Autodesk Fusion 360 part; units mm, degrees
sketch "Sketch3" plane through (0, 0, 0) normal (0, 0, 1) x (1, 0, 0)
  line L0 (90, 40) -> (-90, 40)
  line L1 (-90, 40) -> (-90, -40)
  line L2 (-90, -40) -> (90, -40)
  line L3 (90, -40) -> (90, 40)
  line L4 (90, 40) -> (-90, -40) construction
  line L5 (-90, 40) -> (90, -40) construction
  line L6 (-92, -42) -> (92, -42)
  line L7 (92, -42) -> (92, 42)
  line L8 (92, 42) -> (-92, 42)
  line L9 (-92, 42) -> (-92, -42)
  dimension "d6" = 180
  dimension "d7" = 80
  dimension "d8" = 2
extrude "Extrude2" add sketch "Sketch3" along normal blind 5
extrude "Extrude3" add sketch "Sketch3" along normal blind 4 contours L0 L1 L2 L3
sketch "Sketch6" plane through (0, 0, 5) normal (0, 0, 1) x (-1, 0, 0)
  line L0 (-90, -40) -> (-90, 40)
  line L1 (-90, 40) -> (90, 40)
  line L2 (90, 40) -> (90, -40)
  line L3 (90, -40) -> (-90, -40)
  line L4 (92, -42) -> (92, 42)
  line L5 (92, 42) -> (-92, 42)
  line L6 (-92, 42) -> (-92, -42)
  line L7 (-92, -42) -> (92, -42)
  line L8 (-22, -27) -> (-22, -57)
  line L9 (22, -57) -> (22, -27)
  line L10 (22, -42) -> (-22, -42)
  line L11 (-22, -42) -> (-22, -72)
  line L12 (-22, -72) -> (22, -72)
  line L13 (22, -72) -> (22, -42)
  line L14 (22, -42) -> (-22, -72) construction
  line L15 (-22, -42) -> (22, -72) construction
  point P0 (0, -42)
  point P1 (0, -57)
  dimension "d20" = 44
  dimension "d21" = 30
  dimension "d22" = 44
  dimension "d23" = 30
extrude "Extrude4" add sketch "Sketch6" against normal blind 5 contours L7 L8 L9 L10 L11 L12 L13
sketch "Sketch7" plane through (0, 0, 5) normal (0, 0, 1) x (-1, 0, 0)
  line L0 (-90, -40) -> (-90, 40)
  line L1 (-90, 40) -> (90, 40)
  line L2 (90, 40) -> (90, -40)
  line L3 (90, -40) -> (-90, -40)
  line L4 (92, -42) -> (92, 42)
  line L5 (92, 42) -> (-92, 42)
  line L6 (-92, 42) -> (-92, -42)
  line L7 (-92, -42) -> (-22, -42)
  line L8 (-22, -42) -> (-22, -72)
  line L9 (-22, -72) -> (22, -72)
  line L10 (22, -72) -> (22, -42)
  line L11 (22, -42) -> (92, -42)
  circle A0 centre (-18, -68) radius 1.5
  circle A1 centre (18, -68) radius 1.5
  circle A2 centre (-18, -47) radius 1.5
  circle A3 centre (18, -47) radius 1.5
  dimension "d26" = 3
  dimension "d27" = 4
  dimension "d28" = 4
  dimension "d29" = 3
  dimension "d30" = 3
  dimension "d31" = 3
  dimension "d32" = 4
  dimension "d33" = 4
  dimension "d34" = 4
  dimension "d35" = 7
  dimension "d36" = 4
  dimension "d37" = 7
extrude "Extrude5" cut sketch "Sketch7" against normal blind 6 contours A2
extrude "Extrude6" cut sketch "Sketch7" against normal blind 6 contours A0
extrude "Extrude7" cut sketch "Sketch7" against normal blind 23 contours A3
extrude "Extrude8" cut sketch "Sketch7" against normal blind 15 contours A1
sketch "Sketch8" plane through (0, 0, 4) normal (0, 0, 1) x (-1, 0, 0)
  line L0 (-90, 40) -> (-90, -40)
  line L1 (-90, -40) -> (90, -40)
  line L2 (90, -40) -> (90, 40)
  line L3 (90, 40) -> (-90, 40)
  line L4 (15, 29) -> (-15, 29)
  line L5 (-15, 29) -> (-15, 32)
  line L6 (-15, 32) -> (15, 32)
  line L7 (15, 32) -> (15, 29)
  line L8 (15, 29) -> (-15, 32) construction
  line L9 (-15, 29) -> (15, 32) construction
  circle A0 centre (-13.5, 30.5) radius 1.5
  circle A1 centre (13.5, 30.5) radius 1.5
  circle A2 centre (-11, 35) radius 1
  circle A3 centre (11, 35) radius 1
  point P0 (0, 30.5)
  dimension "d46" = 30
  dimension "d47" = 3
  dimension "d48" = 8
  dimension "d49" = 5
  dimension "d50" = 5
  dimension "d51" = 4
  dimension "d52" = 4
extrude "Extrude9" cut sketch "Sketch8" against normal blind 12 contours L4 L6 A0 A1 | A1 | A0
extrude "Extrude10" cut sketch "Sketch8" against normal blind 25 contours A2 | A3
sketch "Sketch9" plane through (0, 0, 4) normal (0, 0, 1) x (-1, 0, 0)
  circle A0 centre (-11, 35) radius 1
  circle A1 centre (11, 35) radius 1
  line L0 (13.5, 29) -> (-13.5, 29)
  arc A2 (-13.5, 32) -> (-13.5, 29) centre (-13.5, 30.5) ccw
  line L1 (-13.5, 32) -> (13.5, 32)
  arc A3 (13.5, 29) -> (13.5, 32) centre (13.5, 30.5) ccw
  line L2 (-90, 40) -> (-90, -40)
  line L3 (-90, -40) -> (90, -40)
  line L4 (90, -40) -> (90, 40)
  line L5 (90, 40) -> (-90, 40)
  line L6 (70, 24.0265) -> (-70, 24.0265)
  line L7 (0, 24.0265) -> (0, -12)
  line L8 (-70, 24.0265) -> (-15, -12)
  line L9 (15, -12) -> (70, 24.0265)
  line L10 (-15, -12) -> (15, -12)
  line L11 (70, 15) -> (70, -30)
  line L12 (70, -30) -> (50, -30)
  line L13 (70, 15) -> (50, 2)
  line L14 (50, 2) -> (50, -30)
  line L15 (-70, 15) -> (-50, 2)
  line L16 (-70, 15) -> (-70, -30)
  line L17 (-50, 2) -> (-50, -30)
  line L18 (-70, -30) -> (-50, -30)
  point P0 (0, -12)
  dimension "d62" = 28
extrude "Extrude11" cut sketch "Sketch9" against normal blind 25 contours L6 L7 L9 L10 | L6 L7 L8 L10
fillet "Fillet1" radius 1 1 edges at (-70, -24.0265, 2)
fillet "Fillet2" radius 1 3 edges at (70, -24.0265, 2) (15, 12, 2) (-15, 12, 2)
extrude "Extrude12" cut sketch "Sketch9" against normal blind 15 contours L11 L12 L13 L14 | L15 L16 L17 L18
fillet "Fillet3" radius 1 4 edges at (70, -15, 2) (50, -2, 2) (50, 30, 2) (70, 30, 2)
fillet "Fillet4" radius 1 4 edges at (-50, -2, 2) (-70, -15, 2) (-70, 30, 2) (-50, 30, 2)
fillet "Fillet5" radius 1 6 edges at (-22, 72, 2.5) (22, 72, 2.5) (-92, 42, 2.5) (-92, -42, 2.5) (92, 42, 2.5) (92, -42, 2.5)
sketch "Sketch11" plane through (0, 0, 4) normal (0, 0, 1) x (-1, 0, 0)
sketch "Sketch12" plane through (0, 0, 4) normal (0, 0, 1) x (-1, 0, 0)
sketch "Sketch13" plane through (0, 0, 4) normal (0, 0, 1) x (-1, 0, 0)
  circle A0 centre (-11, 35) radius 1.5
  circle A1 centre (11, 35) radius 1.5
  dimension "d79" = 3
  dimension "d80" = 3
extrude "Extrude13" cut sketch "Sketch13" against normal blind 100
The model under review builds one solid part; all positions refer to its coordinate system, in mm. A direction names the side the tool comes from. Round coordinates to 2 decimals unless told otherwise and drop trailing zeros. Loops run counter-clockwise (first coordinate to the right, second up) from the corner with the lowest first, then second, coordinate; pieces in that order, holes last. Notation, with made-up numbers: (-24.5, 26) -> (17.5, 26) arc R14 cw to (17.5, 52) -> close; hole circle Ø8 at (32.25, 23.25). An arc over 180 degrees is marked (long way). Write item = value, one per line. Start each with the question number.
Item 1: Take a section at C-C on z = 2.9. Count the separate pieces of the cut face and the enclosed holes in it, plus the area to 3 significant figures.
Item 2: Take a section at B-B on x = -45.5. Give the boundary of the cut face in (y, z).
Item 3: Take a section at D-D on x = -76. Give the boundary of the cut face in (y, z).
Item 4: Take a section at A-A on x = 2. Give the boundary of the cut face in (y, z).
Item 5: Mouldability with a two-part tool opening along Y and no side actions: class faces 1 (the flat face through (70, 8, 2)), 2 (the flat face through (0, 72, 3)), 3 (the flat face through (92, -1, 2)) as released by +Y, released by -Y, zero draft, split by the parting line, or undercut.
Item 6: For faces 4 (the flat face through (22, 56, 3)), 5 (the flat face through (-1, -42, 2)), 6 (the flat face through (-92, 1, 2)), 7 (the flat face through (-60, 30, 2)), 8 (the flat face through (-56, 42, 2)), list the 3-axis set-ups (+Z, -Z, +X, -X, +Y, -Y) from which the entire face can be reached by the end or side of a thin tool; tool diameter is ignored.
Item 7: To check wall thickness, follow L1, parallel to X at y = 68, z = 2.7; L2, parallel to Y at x = -1.5, z = 0.85; L3, parallel to X at y = 23, z = 0.75. State the ranges of each line that lie inside material, in increasing order.
Item 8: Insertion check: pin 1 (1.5 mm diameter, centred on x = -40, z = 2, fed in from +Y); pin 2 (1 mm diameter, centred on x = -46, y = -30.5, fed in from +Z); pin 3 (2.5 mm diameter, centred on y = 53.5, z = 2.5, fed in from -X). Each pin has a flat end and moves straight along its axis. Give the tip position at first contact, or say it passes through.
Result:
q1.separate_pieces = 1
q1.enclosed_holes = 10
q1.area = 12,000 mm²
q2.outline = (-42, 0) -> (-24.03, 0) -> (-24.03, 4) -> (-40, 4) -> (-40, 5) -> (-42, 5) -> close; (-7.98, 0) -> (42, 0) -> (42, 5) -> (40, 5) -> (40, 4) -> (-7.98, 4) -> close
q3.outline = (-42, 0) -> (42, 0) -> (42, 5) -> (40, 5) -> (40, 4) -> (-40, 4) -> (-40, 5) -> (-42, 5) -> close
q4.outline = (-42, 0) -> (-32, 0) -> (-32, 4) -> (-40, 4) -> (-40, 5) -> (-42, 5) -> close; (-29, 0) -> (-24.03, 0) -> (-24.03, 4) -> (-29, 4) -> close; (12, 0) -> (72, 0) -> (72, 5) -> (40, 5) -> (40, 4) -> (12, 4) -> close
q5.face_1 = undercut
q5.face_2 = released by +Y
q5.face_3 = zero draft
q6.face_4 = +Z, -Z, +X, +Y
q6.face_5 = +Z, -Z, +X, -X, -Y
q6.face_6 = +Z, -Z, -X, +Y, -Y
q6.face_7 = +Z, -Z
q6.face_8 = +Z, -Z, -X, +Y
q7.L1 = -22 to -19.5, -16.5 to 16.5, 19.5 to 22
q7.L2 = -42 to -32, -29 to -24.03, 12 to 72
q7.L3 = -92 to -70, -50 to 50, 70 to 92
q8.pin_1 = 42
q8.pin_2 = 4
q8.pin_3 = -22
